```python
from build123d import *

# Parameters (mm, degrees)
F0_R     = 23
F0_R_2   = 21.5
F1_DEPTH = 1.5
F0_R_3   = 3
F2_DEPTH = 6.5
F3_R     = 1
F4_R     = 1


with BuildPart() as f1:
    # F0 (on Top) → F1 (new body)
    with BuildSketch(Plane.XY):
        with Locations((9.697127, 15.354596)):
            Circle(F0_R)
        with Locations((9.697127, 15.354596)):
            Circle(F0_R_2, mode=Mode.SUBTRACT)
    extrude(amount=F1_DEPTH)

    # F0 (on Top) → F2 (join)
    with BuildSketch(Plane.XY):
        with Locations((9.697127, 15.354596)):
            Circle(F0_R_2)
        with Locations((9.697127, 15.354596)):
            Circle(F0_R_3, mode=Mode.SUBTRACT)
    extrude(amount=F2_DEPTH)

    # F3
    f3_edges = [f1.edges().sort_by_distance(p)[0] for p in [
        (-11.802873, 15.354596, 6.5),
    ]]
    fillet(f3_edges, radius=F3_R)

    # F4
    f4_edges = [f1.edges().sort_by_distance(p)[0] for p in [
        (-13.302873, 15.354596, 0),
    ]]
    fillet(f4_edges, radius=F4_R)


solid = f1.part
```
Read the model definition and answer for the solid it produces. Units are mm, in the model's axes. A direction names the side the tool comes from. Coordinates: 2 decimals unless noted, no trailing zeros. Loops run counter-clockwise (first coordinate to the right, second up) from the corner with the lowest first, then second, coordinate; pieces in that order, holes last. Notation, with made-up numbers: (-29.75, 34) - (11.25, 34) arc R6 ccw to (11.25, 41) - close; hole circle Ø6 at (29.5, 36.25). An arc over 180 degrees is marked (long way). Answer in a Markdown table with one row per item.
1. Determine the mould class of faces 3 (the face through (9, 11, 0)), 4 (the face through (5.036, -5.634, 3.472)), 5 (the face through (6.7, 15.5, 3.2)) for opening direction Y: +Y half, -Y half, draft (parallel to the pull), parting line (faces both ways), or undercut.
Conclusion:
| item | result |
|---|---|
| face 3 | draft |
| face 4 | parting line |
| face 5 | undercut |
2. Straight lines are drawn through the part: line 1 (X direction, y = 14.5, z = 2.25); line 2 (X direction, y = 19, z = 3.25); line 3 (Z direction, x = 28.5, y = 27). For each, find the intervals that lie inside material, in ascending order.
Conclusion:
| item | result |
|---|---|
| line 1 | x = -11.79 to 6.82, 12.57 to 31.18 |
| line 2 | x = -11.49 to 30.89 |
| line 3 | z = 0.01 to 1.5 |
3. Find section A-A, the plane z = 2.5. Write down the section's boundary in (x, y).
Conclusion:
| item | result |
|---|---|
| outline | circle Ø43 at (9.7, 15.35); hole circle Ø6 at (9.7, 15.35) |
4. Given pin 1 (2 mm diameter, centred on y = -1, z = 1, fed in from -X); pin 2 (8 mm diameter, centred on x = -6, y = 21, fed in from -Z); pin 3 (3 mm diameter, centred on x = 2.5, z = 4, fed in from +Y); pin 4 (5 mm diameter, centred on x = 9.7, y = 15.35, fed in from +Z), each flat-ended and moving along its own axis, determine where each tip first touches the part or whether it passes through.
Conclusion:
| item | result |
|---|---|
| pin 1 | stops at x = -7.43 |
| pin 2 | stops at z = 0 |
| pin 3 | stops at y = 36.09 |
| pin 4 | passes through |
5. Which of the six approach directions +Z, -Z, +X, -X, +Y, -Y give full straight-line access (tool end or side, diameter ignored) to faces 1 (the face through (25, 0, 1.5)), 2 (the face through (4.71, -7.1, 1.25))?
Conclusion:
| item | result |
|---|---|
| face 1 | +Z |
| face 2 | +Z, -Z |
